Geometry check sheet. Reference: the model listing, model coordinates, mm. A direction names the side the tool comes from. Round coordinates to 2 decimals unless told otherwise and drop trailing zeros. Write each loop counter-clockwise with the first axis right and the second up, starting at its lowest first coordinate (ties: lowest second). Pieces come first, ordered by that corner, then holes. Notation, with made-up numbers: (-26.75, 65.5) - (-3.75, 65.5) arc R18 ccw to (-3.75, 88.5) - close; hole circle Ø4 at (25, 22). An arc over 180 degrees is marked (long way). One line per question, with ' | ' between items. Start each with the question number.
from build123d import *

# Parameters (mm, degrees)
F1_DEPTH = 41.275
F4_D     = 14.2875
F7_D     = 14.2875


# Not quite as in the source:
# - a length typed as a fraction of an inch, garbled in the dataset ("3 / 203.2 mm" for 3/8 in), is restored


with BuildPart() as f1:
    # F0 (on Top) → F1 (new body)
    with BuildSketch(Plane.XY):
        with BuildLine():
            ThreePointArc((10.31875, 97.63125), (3.0222919016, 94.6089580984), (0, 87.3125))
            Line((0, 87.3125), (0, 0))
            Line((0, 0), (6.35, 0))
            Line((6.35, 0), (6.35, 87.3125))
            ThreePointArc((6.35, 87.3125), (7.5124199622, 90.1188300378), (10.31875, 91.28125))
            Line((10.31875, 91.28125), (97.63125, 91.28125))
            Line((97.63125, 91.28125), (97.63125, 97.63125))
            Line((97.63125, 97.63125), (10.31875, 97.63125))
        make_face()
    extrude(amount=F1_DEPTH)

    # F4 (through all)
    with Locations(Plane.YZ.offset(6.35)):
        with Locations((20.6375, 20.6375), (68.2625, 20.6375)):
            Hole(F4_D / 2)

    # F7 (through all)
    with Locations(Plane.XZ.offset(-91.28125)):
        with Locations((29.36875, 20.6375), (76.99375, 20.6375)):
            Hole(F7_D / 2)


solid = f1.part
Q1. Section check B-B, the plane y = 68. Record the cut outline in (x, z) (3 decimals), then the cut area to 3 significant figures.
Q2. Set-up check for faces 1 (the flat face through (53, 91.281, 20)), 2 (the cylindrical face through (70.395, 94.501, 17.901)): record each of +Z, -Z, +X, -X, +Y, -Y from which the full face is reachable in a straight line by a thin tool's end or side.
Q3. Section check A-A, the plane z = 23.5. Record the cut outline in (x, y).
Q4. Draft check along Y on faces 3 (the cylindrical face through (7.482, 90.088, 20.349)), 4 (the flat face through (0, 44, 20)), 5 (the cylindrical face through (3.131, 61.663, 17.901)), 6 (the cylindrical face through (3.13, 17.34, 14.3)). Enter one of: pulls with the +Y half, pulls with the -Y half, needs draft (parallel to the pull), parting line crosses it, or undercut.
Q5. Go/stop test with flat-tipped pins: P1, Ø13, axis at y = 20.64, z = 20.64, coming from the -X side; P2, Ø18.5, axis at x = 29.37, z = 20.64, coming from the -Y side; P3, Ø20.5, axis at y = 50, z = 12.5, coming from the +X side. Record where each tip stops, or that it passes through.
Q6. Thickness scan on line 1 (Y direction, x = 64, z = 5.5); line 2 (X direction, y = 85, z = 37.5). Record the ranges inside material, lowest first.
Q7. Section check D-D, the plane z = 34.5. Record the cut outline in (x, y).
Q8. Section check C-C, the plane x = 35. Record the cut outline in (y, z) (3 decimals).
Result sheet:
1) outline: (0, 0) - (6.35, 0) - (6.35, 13.499) - (0, 13.499) - close; (0, 27.776) - (6.35, 27.776) - (6.35, 41.275) - (0, 41.275) - close | area: 171 mm²
2) face 1: +Z, -Z, +X, -Y | face 2: +Y, -Y
3) outline: (0, 0) - (6.35, 0) - (6.35, 14.09) - (0, 14.09) - close; (0, 27.18) - (6.35, 27.18) - (6.35, 61.72) - (0, 61.72) - close; (0, 74.81) - (6.35, 74.81) - (6.35, 87.31) arc R3.97 cw to (10.32, 91.28) - (22.82, 91.28) - (22.82, 97.63) - (10.32, 97.63) arc R10.32 ccw to (0, 87.31) - close; (35.91, 91.28) - (70.45, 91.28) - (70.45, 97.63) - (35.91, 97.63) - close; (83.54, 91.28) - (97.63, 91.28) - (97.63, 97.63) - (83.54, 97.63) - close
4) face 3: pulls with the -Y half | face 4: needs draft | face 5: undercut | face 6: undercut
5) P1: through | P2: y = 91.28 | P3: x = 6.35
6) line 1: 91.28 to 97.63 | line 2: 0 to 6.35
7) outline: (0, 0) - (6.35, 0) - (6.35, 87.31) arc R3.97 cw to (10.32, 91.28) - (97.63, 91.28) - (97.63, 97.63) - (10.32, 97.63) arc R10.32 ccw to (0, 87.31) - close
8) outline: (91.281, 0) - (97.631, 0) - (97.631, 16.242) - (91.281, 16.242) - close; (91.281, 25.033) - (97.631, 25.033) - (97.631, 41.275) - (91.281, 41.275) - close
